Here's how the part is built. I have some questions about the finished solid (model axes, mm). A direction names the side the tool comes from. Coordinates: 2 decimals unless noted, no trailing zeros. Loops run counter-clockwise (first coordinate to the right, second up) from the corner with the lowest first, then second, coordinate; pieces in that order, holes last. Notation, with made-up numbers: (79, 48) -> (90, 48) arc R18 ccw to (90, 68) -> close; hole circle Ø10 at (-18, 41). An arc over 180 degrees is marked (long way). Answer as a JSON object with one key per item and string values. Group by question number.
Q1. I'm going to push flat-ended pins straight in: pin 1 (10 mm diameter, centred on x = -1, y = 1, fed in from +Z); pin 2 (5.5 mm diameter, centred on x = -3, z = 3, fed in from -Y); pin 3 (3 mm diameter, centred on x = -3.5, y = 3.5, fed in from -Z); pin 4 (7 mm diameter, centred on x = -1.5, z = -6.5, fed in from +Y). Where does each tip first touch, or does it pass through?
Q2. I want a section at D-D on x = 7.5. Write out the boundary of the cut face in (y, z), then the cut area to 3 significant figures.
Q3. I want a section at B-B on z = 0.5. Write out the boundary of the cut face in (x, y).
Q4. Thinking about a two-plate mould opening in Z: for faces 6 (the flat face through (-10, -4, -3)), 7 (the flat face through (0, -6, -9.1)), 8 (the cylindrical face through (-10.64, -7.64, -11.7)), which applies, released by +Z, released by -Z, zero draft, split by the parting line, or undercut?
Q5. I need wall thicknesses on line 1 (Z direction, x = 0, y = -7.8); line 2 (X direction, y = -7.9, z = -6.3); line 3 (X direction, y = 5.75, z = 4.5). Which ranges of each line are inside material? Lowest first, please.
Q6. On a 3-axis mill with a long thin cutter (end or side, diameter ignored), from which of +Z, -Z, +X, -X, +Y, -Y can I reach the whole of each face in a straight line? I mean faces 1 (the flat face through (0, -6, -3.5)), 2 (the flat face through (-10.76, -1.938, -5.205)), 3 (the flat face through (0, -1, 1)), 4 (the flat face through (0, 7, 4)), 5 (the flat face through (-3.707, -5.521, -8.48)). Say none if no direction works.
Q7. I want a section at A-A on x = 0. Write out the boundary of the cut face in (y, z), then the cut area to 4 significant figures.
Q8. I want a section at C-C on y = 5.5. Write out the boundary of the cut face in (x, z), then the cut area to 3 significant figures.
```python
from build123d import *

# Parameters (mm, degrees)
SKETCH_1_W                  = 23
SKETCH_1_H                  = 17
EXTRUDE_1_DEPTH             = 6.5
SKETCH_2_W                  = 20
SKETCH_2_H                  = 15.5
CUT_EXTRUDE_1_DEPTH         = 5
SKETCH_3_W                  = 23
SKETCH_3_H                  = 1.5
EXTRUDE_2_DEPTH             = 12.6
EXTRUDE_3_DEPTH             = 3
EXTRUDE_6_REACH             = 21.397
SKETCH_7_W                  = 1.5
SKETCH_7_H                  = 7.259859141
EXTRUDE_6_DIRECTION_2_REACH = 21.397
HOLE_WIZARD_M3_1_D          = 3.2
FILLET_1_R                  = 3
CUT_EXTRUDE_2_REACH         = 21.059
SKETCH_10_W                 = 6
SKETCH_10_H                 = 3.5


with BuildPart() as part:
    # 草图1 → 凸台-拉伸1 (new body)
    with BuildSketch(Plane.XY):
        Rectangle(SKETCH_1_W, SKETCH_1_H)
    extrude(amount=EXTRUDE_1_DEPTH)

    # 草图2 → 切除-拉伸1 (cut)
    with BuildSketch(Plane.XY.offset(6.5)):
        with Locations((0, -0.75)):
            Rectangle(SKETCH_2_W, SKETCH_2_H)
    extrude(amount=-CUT_EXTRUDE_1_DEPTH, mode=Mode.SUBTRACT)

    # 草图3 → 凸台-拉伸2 (add)
    with BuildSketch(Plane(origin=(0, 0, 0), x_dir=(-1, 0, 0), z_dir=(0, 0, -1))):
        with Locations((0, -7.75)):
            Rectangle(SKETCH_3_W, SKETCH_3_H)
    extrude(amount=EXTRUDE_2_DEPTH)

    # 草图4 → 凸台-拉伸3 (add)
    with BuildSketch(Plane(origin=(0, -7, 0), x_dir=(1, 0, 0), z_dir=(0, 1, 0))):
        Polygon((4.965212315, 6.3), (2.482606158, 10.6), (-2.482606158, 10.6), (-4.965212315, 6.3), (-2.482606158, 2), (2.482606158, 2), align=None)
        Polygon((3.233161507, 6.3), (1.616580754, 9.1), (-1.616580754, 9.1), (-3.233161507, 6.3), (-1.616580754, 3.5), (1.616580754, 3.5), align=None, mode=Mode.SUBTRACT)
    extrude(amount=EXTRUDE_3_DEPTH)

    # 凸台-拉伸6: up to this face of the body (flat: up to its plane)
    extrude_6_end = Plane(part.part.faces().sort_by_distance((0, -7, -6.3))[0])
    # 草图7 → 凸台-拉伸6 (add, up to the picked face)
    with BuildSketch(Plane(origin=(0, -3.5, -3.5), x_dir=(-1, 0, 0), z_dir=(0, -0.7071067811865475, -0.7071067811865477)), mode=Mode.PRIVATE) as extrude_6_sk1:
        with Locations((-10.75, -1.319817897)):
            Rectangle(SKETCH_7_W, SKETCH_7_H)
    extrude_6_tool1 = split(extrude(extrude_6_sk1.sketch, amount=EXTRUDE_6_REACH, mode=Mode.PRIVATE), bisect_by=extrude_6_end, keep=Keep.BOTH, mode=Mode.PRIVATE)
    extrude_6 = extrude_6_tool1.solids().sort_by(Axis((10.75, -4.433252, -2.566748), (0, -0.7071067811865475, -0.7071067811865477)))[0]
    add(extrude_6)

    # 凸台-拉伸6 direction 2: up to this face of the body (flat: up to its plane)
    extrude_6_direction_2_end = Plane(part.part.faces().sort_by_distance((0, 0.75, 0))[0])
    # 草图7 → 凸台-拉伸6 direction 2 (add, up to the picked face)
    with BuildSketch(Plane(origin=(0, -3.5, -3.5), x_dir=(-1, 0, 0), z_dir=(0, -0.7071067811865475, -0.7071067811865477)), mode=Mode.PRIVATE) as extrude_6_direction_2_sk1:
        with Locations((-10.75, -1.319817897)):
            Rectangle(SKETCH_7_W, SKETCH_7_H)
    extrude_6_direction_2_tool1 = split(extrude(extrude_6_direction_2_sk1.sketch, amount=-EXTRUDE_6_DIRECTION_2_REACH, mode=Mode.PRIVATE), bisect_by=extrude_6_direction_2_end, keep=Keep.BOTH, mode=Mode.PRIVATE)
    extrude_6_direction_2 = extrude_6_direction_2_tool1.solids().sort_by(Axis((10.75, -4.433252, -2.566748), (0, 0.7071067811865475, 0.7071067811865477)))[0]
    add(extrude_6_direction_2)

    # 镜向1: 凸台-拉伸6, 凸台-拉伸6 direction 2 across plane
    add(extrude_6.mirror(Plane(origin=(0, 0, 0), x_dir=(0, 0, 1), z_dir=(1, 0, 0))))
    add(extrude_6_direction_2.mirror(Plane(origin=(0, 0, 0), x_dir=(0, 0, 1), z_dir=(1, 0, 0))))

    # M3 间隙孔1 (through all)
    with Locations(Plane(origin=(0, -7, 0), x_dir=(1, 0, 0), z_dir=(0, 1, 0))):
        with Locations((0, 6.3)):
            Hole(HOLE_WIZARD_M3_1_D / 2)

    # 圆角1
    fillet_1_edges = [part.edges().sort_by_distance(p)[0] for p in [
        (-11.5, -7.75, -12.6),
        (11.5, -7.75, -12.6),
    ]]
    fillet(fillet_1_edges, radius=FILLET_1_R)

    # 草图10 → 切除-拉伸2 (cut, up to next)
    with BuildSketch(Plane(origin=(0, 0, 0), x_dir=(-1, 0, 0), z_dir=(0, 0, -1)), mode=Mode.PRIVATE) as cut_extrude_2_sk1:
        with Locations((0, -2.75)):
            Rectangle(SKETCH_10_W, SKETCH_10_H)
    cut_extrude_2_tool1 = extrude(cut_extrude_2_sk1.sketch, amount=-CUT_EXTRUDE_2_REACH, mode=Mode.PRIVATE) & part.part
    add(cut_extrude_2_tool1.solids().sort_by_distance((0, -2.75, 0))[0], mode=Mode.SUBTRACT)


solid = part.part
```
Result set:
{
 "1": {"pin 1": "stops at z = 1.5", "pin 2": "stops at y = -8.5", "pin 3": "stops at z = 0", "pin 4": "stops at y = -4"},
 "2": {"outline": "(-8.5, -12.6) -> (-7, -12.6) -> (-7, 0) -> (8.5, 0) -> (8.5, 6.5) -> (7, 6.5) -> (7, 1.5) -> (-8.5, 1.5) -> close", "area": "51.9 mm²"},
 "3": {"outline": "(-11.5, -8.5) -> (11.5, -8.5) -> (11.5, 8.5) -> (-11.5, 8.5) -> close; hole (-3, -4.5) -> (3, -4.5) -> (3, -1) -> (-3, -1) -> close"},
 "4": {"face 6": "zero draft", "face 7": "undercut", "face 8": "released by -Z"},
 "5": {"line 1": "z = -12.6 to -7.9, -4.7 to 1.5", "line 2": "x = -11.5 to -1.6, 1.6 to 11.5", "line 3": "x = -11.5 to -10, 10 to 11.5"},
 "6": {"face 1": "+Y", "face 2": "-Z, -X, +Y", "face 3": "+Z, -Z", "face 4": "+Z, -Y", "face 5": "-Z, +Y"},
 "7": {"outline": "(-8.5, -12.6) -> (-7, -12.6) -> (-7, -10.6) -> (-4, -10.6) -> (-4, -9.1) -> (-7, -9.1) -> (-7, -7.9) -> (-8.5, -7.9) -> close; (-8.5, -4.7) -> (-7, -4.7) -> (-7, -3.5) -> (-4, -3.5) -> (-4, -2) -> (-7, -2) -> (-7, 0) -> (-4.5, 0) -> (-4.5, 1.5) -> (-8.5, 1.5) -> close; (-1, 0) -> (8.5, 0) -> (8.5, 6.5) -> (7, 6.5) -> (7, 1.5) -> (-1, 1.5) -> close", "area": "50.85 mm²"},
 "8": {"outline": "(-11.5, 0) -> (11.5, 0) -> (11.5, 6.5) -> (10, 6.5) -> (10, 1.5) -> (-10, 1.5) -> (-10, 6.5) -> (-11.5, 6.5) -> close", "area": "49.5 mm²"}
}
